Design review of the part built by this model. Coordinates are the model's own, in mm. Give positions to 0.01 mm unless a question says otherwise; leave off trailing zeros. Order: outer loops, then holes, each group sorted by start corner. A loop starts at its lowest first (then second) coordinate and runs counter-clockwise, first axis right, second up. Notation, with made-up numbers: (23.5, 88.25) -> (60.5, 88.25) arc R24 cw to (60.5, 121.25) -> close; hole circle Ø6 at (-22, -33). An arc over 180 degrees is marked (long way). One line per item, written item: value. Start each with the question number.
1) Consider section A-A (x = -24.5). State the section outline as (y, z) points, plus the area to 3 significant figures.
2) Wall thickness on line 1 along Z through (x, y) = (20.5, 1.2); line 2 along X through (y, z) = (0.6, 16); line 3 along Z through (x, y) = (-15, 0.6): over which ranges is each line inside the solid? List them lowest first. Write a range as from..to.
3) Consider section C-C (z = 5.5). State the section outline as (x, y) points, plus the area to 3 significant figures.
4) Consider section D-D (x = 27.5). State the section outline as (y, z) points.
5) Consider section B-B (y = 1.1). State the section outline as (x, z) points.
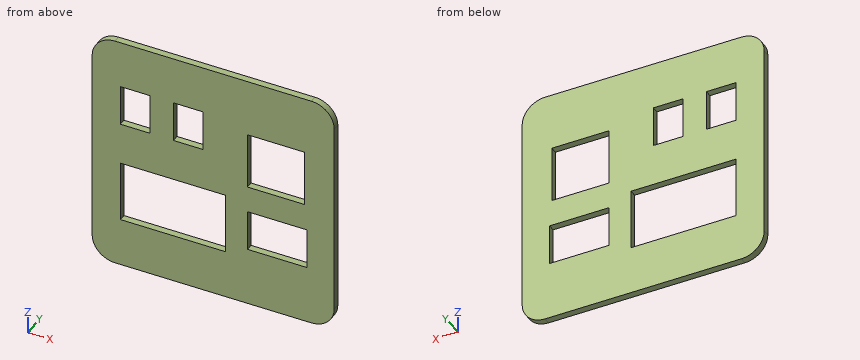
from build123d import *

# Parameters (mm, degrees)
SKETCH1_W           = 25
SKETCH1_H           = 25
SKETCH1_W_2         = 26
SKETCH1_H_2         = 18
SKETCH1_W_3         = 46
SKETCH1_H_3         = 27
SKETCH1_W_4         = 13
BOSS_EXTRUDE1_DEPTH = 3


with BuildPart() as part:
    # Sketch1 → Boss-Extrude1 (new body)
    with BuildSketch(Plane(origin=(0, 0, 0), x_dir=(1, 0, 0), z_dir=(0, 1, 0))):
        with BuildLine():
            ThreePointArc((43, 53), (50.071067812, 50.071067812), (53, 43))
            Line((53, 43), (53, -43))
            ThreePointArc((53, -43), (50.071067812, -50.071067812), (43, -53))
            Line((43, -53), (-43, -53))
            ThreePointArc((-43, -53), (-50.071067812, -50.071067812), (-53, -43))
            Line((-53, -43), (-53, 43))
            ThreePointArc((-53, 43), (-50.071067812, 50.071067812), (-43, 53))
            Line((-43, 53), (43, 53))
        make_face()
        with BuildLine():
            Line((-40, 50), (40, 50))
            ThreePointArc((40, 50), (47.071067812, 47.071067812), (50, 40))
            Line((50, 40), (50, -40))
            ThreePointArc((50, -40), (47.071067812, -47.071067812), (40, -50))
            Line((40, -50), (-40, -50))
            ThreePointArc((-40, -50), (-47.071067812, -47.071067812), (-50, -40))
            Line((-50, -40), (-50, 40))
            ThreePointArc((-50, 40), (-47.071067812, 47.071067812), (-40, 50))
        make_face(mode=Mode.SUBTRACT)
        with BuildLine():
            ThreePointArc((40, 50), (47.071067812, 47.071067812), (50, 40))
            Line((50, 40), (50, -40))
            ThreePointArc((50, -40), (47.071067812, -47.071067812), (40, -50))
            Line((40, -50), (-40, -50))
            ThreePointArc((-40, -50), (-47.071067812, -47.071067812), (-50, -40))
            Line((-50, -40), (-50, 40))
            ThreePointArc((-50, 40), (-47.071067812, 47.071067812), (-40, 50))
            Line((-40, 50), (40, 50))
        make_face()
        with Locations((27.5, -15.109148856)):
            Rectangle(SKETCH1_W, SKETCH1_H, mode=Mode.SUBTRACT)
        with Locations((28, 18.185109271)):
            Rectangle(SKETCH1_W_2, SKETCH1_H_2, mode=Mode.SUBTRACT)
        with Locations((-17.665765758, 18.038886372)):
            Rectangle(SKETCH1_W_3, SKETCH1_H_3, mode=Mode.SUBTRACT)
        with Locations((-34.165765758, -23.046005222)):
            Rectangle(SKETCH1_W_4, SKETCH1_H_2, mode=Mode.SUBTRACT)
        with Locations((-10.934651265, -23.046005222)):
            Rectangle(SKETCH1_W_4, SKETCH1_H_2, mode=Mode.SUBTRACT)
    extrude(amount=BOSS_EXTRUDE1_DEPTH)


solid = part.part
Checked values:
1. outline: (0, -53) -> (3, -53) -> (3, -31.54) -> (0, -31.54) -> close; (0, -4.54) -> (3, -4.54) -> (3, 53) -> (0, 53) -> close
1. area: 237 mm^2
2. line 1: z = -53..-27.19, -9.19..2.61, 27.61..53
2. line 2: x = -53..-40.67, -27.67..-17.43, -4.43..15, 40..53
2. line 3: z = -53..-31.54, -4.54..14.05, 32.05..53
3. outline: (-53, 0) -> (15, 0) -> (15, 3) -> (-53, 3) -> close; (40, 0) -> (53, 0) -> (53, 3) -> (40, 3) -> close
3. area: 243 mm^2
4. outline: (0, -53) -> (3, -53) -> (3, -27.19) -> (0, -27.19) -> close; (0, -9.19) -> (3, -9.19) -> (3, 2.61) -> (0, 2.61) -> close; (0, 27.61) -> (3, 27.61) -> (3, 53) -> (0, 53) -> close
5. outline: (-53, -43) arc R10 ccw to (-43, -53) -> (43, -53) arc R10 ccw to (53, -43) -> (53, 43) arc R10 ccw to (43, 53) -> (-43, 53) arc R10 ccw to (-53, 43) -> close; hole (-40.67, -31.54) -> (5.33, -31.54) -> (5.33, -4.54) -> (-40.67, -4.54) -> close; hole (-40.67, 14.05) -> (-27.67, 14.05) -> (-27.67, 32.05) -> (-40.67, 32.05) -> close; hole (-17.43, 14.05) -> (-4.43, 14.05) -> (-4.43, 32.05) -> (-17.43, 32.05) -> close; hole (15, -27.19) -> (41, -27.19) -> (41, -9.19) -> (15, -9.19) -> close; hole (15, 2.61) -> (40, 2.61) -> (40, 27.61) -> (15, 27.61) -> close
